```python
from build123d import *

# Parameters (mm, degrees)
SKETCH1_R           = 4.7625
EXTRUDE1_DEPTH      = 15.875
SKETCH2_R           = 6.477
EXTRUDE2_DEPTH      = 3.302
CHAMFER1_SIZE       = 0.6604
SKETCH3_R           = 1.984375
EXTRUDE3_DEPTH      = 7.477
EXTRUDE3_DEPTH_BACK = 7.477
CHAMFER2_SIZE       = 0.47625


with BuildPart() as part:
    # Sketch1 → Extrude1 (new body, symmetric)
    with BuildSketch(Plane.XY):
        Circle(SKETCH1_R)
    extrude(amount=EXTRUDE1_DEPTH, both=True)

    # Sketch2 → Extrude2 (add)
    with BuildSketch(Plane.XY.offset(15.875)):
        Circle(SKETCH2_R)
    extrude(amount=EXTRUDE2_DEPTH)

    # Chamfer1
    chamfer1_edges = [part.edges().sort_by_distance(p)[0] for p in [
        (-6.477, 0, 19.177),
    ]]
    chamfer(chamfer1_edges, length=CHAMFER1_SIZE)

    # Sketch3 → Extrude3 (cut, two sides)
    with BuildSketch(Plane(origin=(0, 0, 0), x_dir=(0, 0, -1), z_dir=(1, 0, 0))) as extrude3_sk:
        with Locations((11.509375, 0)):
            Circle(SKETCH3_R)
    extrude(amount=EXTRUDE3_DEPTH, mode=Mode.SUBTRACT)
    extrude(extrude3_sk.sketch, amount=-EXTRUDE3_DEPTH_BACK, mode=Mode.SUBTRACT)

    # Chamfer2
    chamfer2_edges = [part.edges().sort_by_distance(p)[0] for p in [
        (-4.7625, 0, -15.875),
    ]]
    chamfer(chamfer2_edges, length=CHAMFER2_SIZE)


solid = part.part
```
The listing builds one solid part. Answer for the finished solid, in the listing's coordinates (mm). A direction names the side the tool comes from. Give positions to 0.01 mm unless a question says otherwise; leave off trailing zeros. Loops run counter-clockwise (first coordinate to the right, second up) from the corner with the lowest first, then second, coordinate; pieces in that order, holes last. Notation, with made-up numbers: (-5, 16.25) - (34, 16.25) arc R4 ccw to (34, 21.25) - close; hole circle Ø11 at (70.25, 59.5). An arc over 180 degrees is marked (long way). Return JSON: item names as keys, results as strings. Group by question number.
1. Find section A-A (y = 0). Write down the section's boundary in (x, z) (1 decimal).
2. Straight lines are drawn through the part: line 1 (Z direction, x = -1.65, y = 0) (3 decimals); line 2 (Y direction, x = 0, z = -1); line 3 (Z direction, x = -1.5, y = 0.5) (3 decimals). For each, find the intervals that lie inside material, in ascending order. Write a range as [from, to].
3. Find section B-B (z = 4). Write down the section's boundary in (x, y) (1 decimal).
4. Which of the six approach directions +Z, -Z, +X, -X, +Y, -Y give full straight-line access (tool end or side, diameter ignored) to faces 1 (the flat face through (0, 0, 19.177)), 2 (the flat face through (0, 5, 15.875))?
5. Given pin 1 Ø5 at (y, z) = (0.5, 10) entering from -X; pin 2 Ø1 at (x, z) = (2, 9.5) entering from -Y; pin 3 Ø2.5 at (y, z) = (0, -11.51) entering from -X; pin 4 Ø4 at (x, y) = (2.5, -4.5) entering from -Z (3 decimals), each flat-ended and moving along its own axis, determine where each tip first touches the part or whether it passes through.
Verdict:
{
 "1": {"outline": "(-6.5, 15.9) - (-4.8, 15.9) - (-4.8, -9.5) - (4.8, -9.5) - (4.8, 15.9) - (6.5, 15.9) - (6.5, 18.5) - (5.8, 19.2) - (-5.8, 19.2) - (-6.5, 18.5) - close; (-4.8, -15.4) - (-4.3, -15.9) - (4.3, -15.9) - (4.8, -15.4) - (4.8, -13.5) - (-4.8, -13.5) - close"},
 "2": {"line 1": "z = [-15.875, -13.494], [-9.525, 19.177]", "line 2": "y = [-4.76, 4.76]", "line 3": "z = [-15.875, -13.43], [-9.589, 19.177]"},
 "3": {"outline": "circle Ø9.5 at (0, 0)"},
 "4": {"face 1": "+Z, +X, -X, +Y, -Y", "face 2": "-Z"},
 "5": {"pin 1": "stops at x = -4.76", "pin 2": "stops at y = -4.52", "pin 3": "passes through", "pin 4": "stops at z = -15.875"}
}
